Design review of the part built by this model. Coordinates are the model's own, in mm. Face numbers are marked on the shaded views. A direction names the side the tool comes from. Coordinates: 2 decimals unless noted, no trailing zeros. Write each loop counter-clockwise with the first axis right and the second up, starting at its lowest first coordinate (ties: lowest second). Pieces come first, ordered by that corner, then holes.
Q1. For the marked faces 1 and 2, list the 3-axis set-ups (+Z, -Z, +X, -X, +Y, -Y) from which the entire face can be reached by the end or side of a thin tool; tool diameter is ignored.
Q2. Take a section at D-D, the plane z = 2.1. Write out the cut boundary in (x, y).
Q3. Take a section at A-A, the plane x = 0. Write out the cut boundary in (y, z), plus the area to 3 significant figures.
Q4. Take a section at C-C, the plane x = 1.5. Write out the cut boundary in (y, z), plus the area to 3 significant figures.
Q5. For L1, parallel to Y at x = 0, z = 1.95; L2, parallel to Y at x = 0, z = 0.8; L3, parallel to Z at x = -0.5, y = 14.5, list the stretches that pass through material, from the lowest coordinate up.
Q6. For pin 1 Ø1.5 at (x, y) = (-1, 14) entering from +Z; pin 2 Ø1.5 at (y, z) = (5.5, 0.5) entering from -X, all flat-tipped, find the tip position at first contact; note any pin that passes through.
Q7. The part is to be moulded in two halves that separate along X. For the marked faces 3, 4 and 5, say which applies: released by +X, released by -X, zero draft, split by the parting line, or undercut.
Q8. Take a section at B-B, the plane z = 0.3. Write out the cut boundary in (x, y), plus the area to 3 significant figures.
from build123d import *

# Parameters (mm, degrees)
F1_DEPTH = 1.5
F0_R     = 2
F2_DEPTH = 4


with BuildPart() as f1:
    # F0 (on Top) → F1 (new body)
    with BuildSketch(Plane.XY):
        with BuildLine():
            ThreePointArc((2, 14.5), (0, 16.5), (-2, 14.5))
            ThreePointArc((-2, 14.5), (0, 12.5), (2, 14.5))
        make_face()
        with BuildLine():
            Line((-2, 14.5), (-3.4258823529, 0.7164705882))
            ThreePointArc((-3.4258823529, 0.7164705882), (0, 3.5), (3.4258823529, 0.7164705882))
            Line((3.4258823529, 0.7164705882), (2, 14.5))
            ThreePointArc((2, 14.5), (0, 12.5), (-2, 14.5))
        make_face()
    extrude(amount=F1_DEPTH)

    # F0 (on Top) → F2 (join)
    with BuildSketch(Plane.XY):
        with BuildLine():
            Line((-3.4258823529, 0.7164705882), (-3.5, 0))
            ThreePointArc((-3.5, 0), (0, -3.5), (3.5, 0))
            Line((3.5, 0), (3.4258823529, 0.7164705882))
            ThreePointArc((3.4258823529, 0.7164705882), (0, 3.5), (-3.4258823529, 0.7164705882))
        make_face()
        Circle(F0_R, mode=Mode.SUBTRACT)
    extrude(amount=F2_DEPTH)


solid = f1.part
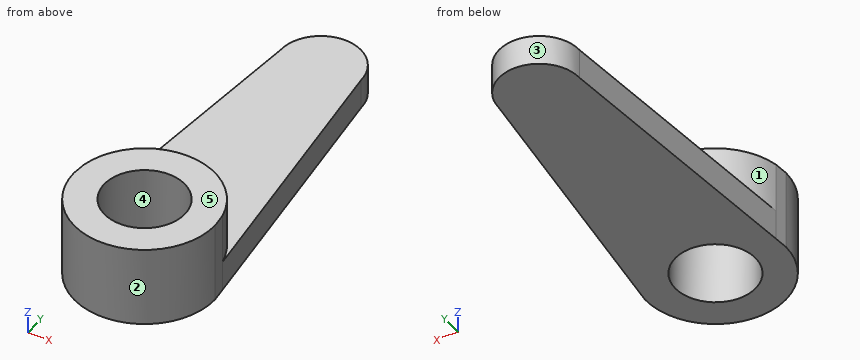
Responses:
1. face 1: +Z, +Y
1. face 2: +Z, -Z, -Y
2. outline: (-3.5, 0) arc R3.5 ccw to (3.5, 0) - (3.43, 0.72) arc R3.5 ccw to (-3.43, 0.72) - close; hole circle Ø4 at (0, 0)
3. outline: (-3.5, 0) - (-2, 0) - (-2, 4) - (-3.5, 4) - close; (2, 0) - (16.5, 0) - (16.5, 1.5) - (3.5, 1.5) - (3.5, 4) - (2, 4) - close
3. area: 31.5 mm2
4. outline: (-3.16, 0) - (-1.32, 0) - (-1.32, 4) - (-3.16, 4) - close; (1.32, 0) - (15.82, 0) - (15.82, 1.5) - (3.16, 1.5) - (3.16, 4) - (1.32, 4) - close
4. area: 33.7 mm2
5. L1: y = -3.5 to -2, 2 to 3.5
5. L2: y = -3.5 to -2, 2 to 16.5
5. L3: z = 0 to 1.5
6. pin 1: stops at z = 1.5
6. pin 2: stops at x = -3.01
7. face 3: split by the parting line
7. face 4: undercut
7. face 5: zero draft
8. outline: (-3.5, 0) arc R3.5 ccw to (3.5, 0) - (2, 14.5) arc R2 ccw to (-2, 14.5) - close; hole circle Ø4 at (0, 0)
8. area: 92.7 mm2
